Geometry check sheet. Reference: the model listing, model coordinates, mm. A direction names the side the tool comes from. Round coordinates to 2 decimals unless told otherwise and drop trailing zeros. Order: outer loops, then holes, each group sorted by start corner. A loop starts at its lowest first (then second) coordinate and runs counter-clockwise, first axis right, second up.
```python
from build123d import *

# Parameters (mm, degrees)
SKETCH_1_R                   = 7
EXTRUDE_1_DEPTH              = 10
SKETCH_2_R                   = 8
EXTRUDE_2_DEPTH              = 4
SKETCH_3_R                   = 3
EXTRUDE_3_DEPTH              = 9.5
CUT_EXTRUDE_1_DEPTH          = 28.367864531
CUT_EXTRUDE_1_DEPTH_BACK     = 28.367864531
SKETCH_4_R                   = 1
SKETCH_8_R                   = 1
EXTRUDE_4_DEPTH              = 2
HOLE_WIZARD_M5_1_D           = 5.5
HOLE_WIZARD_M5_1_CBORE_D     = 11
HOLE_WIZARD_M5_1_CBORE_DEPTH = 6.5
FILLET_1_R                   = 2


with BuildPart() as part:
    # 草图1 → 凸台-拉伸1 (new body)
    with BuildSketch(Plane(origin=(0, 0, 0), x_dir=(1, 0, 0), z_dir=(0, 1, 0))):
        with Locations(Location((0, 0, 0), (0, 0, 270))):
            Circle(SKETCH_1_R)
    extrude(amount=EXTRUDE_1_DEPTH)

    # 草图2 → 凸台-拉伸2 (add)
    with BuildSketch(Plane(origin=(0, 10, 0), x_dir=(1, 0, 0), z_dir=(0, 1, 0))):
        with Locations(Location((0, 0, 0), (0, 0, 270))):
            Circle(SKETCH_2_R)
    extrude(amount=EXTRUDE_2_DEPTH)

    # 草图3 → 凸台-拉伸3 (add, symmetric)
    with BuildSketch(Plane(origin=(0, 0, 0), x_dir=(0, 0, -1), z_dir=(1, 0, 0))):
        with Locations((0, 15)):
            Circle(SKETCH_3_R)
    extrude(amount=EXTRUDE_3_DEPTH, both=True)

    # 草图4 → 切除-拉伸1 (cut, two sides: drawn at the far end of the back side and taken through both)
    with BuildSketch(Plane(origin=(9.5, 0, 0), x_dir=(0, 0, -1), z_dir=(1, 0, 0)).offset(-CUT_EXTRUDE_1_DEPTH_BACK)):
        with Locations((0, 15)):
            Circle(SKETCH_4_R)
    extrude(amount=CUT_EXTRUDE_1_DEPTH + CUT_EXTRUDE_1_DEPTH_BACK, mode=Mode.SUBTRACT)

    # 草图8 → 凸台-拉伸4 (add, symmetric)
    with BuildSketch(Plane(origin=(0, 0, 0), x_dir=(0, 0, -1), z_dir=(1, 0, 0))):
        Polygon((0, 0), (-20.85568787, 17.5), (-32, 17.5), (-32, 22.5), (-19, 22.5), (0, 7.5), align=None)
        with Locations((-30, 20)):
            Circle(SKETCH_8_R, mode=Mode.SUBTRACT)
        with Locations((-25, 20)):
            Circle(SKETCH_8_R, mode=Mode.SUBTRACT)
    extrude(amount=EXTRUDE_4_DEPTH, both=True)

    # M5 六角头螺栓的柱形沉头孔1 (through all)
    with Locations(Plane(origin=(0, 0, 0), x_dir=(-1, 0, 0), z_dir=(0, -1, 0))):
        with Locations((0, 0)):
            CounterBoreHole(HOLE_WIZARD_M5_1_D / 2, HOLE_WIZARD_M5_1_CBORE_D / 2, HOLE_WIZARD_M5_1_CBORE_DEPTH)

    # 圆角1
    fillet_1_edges = [part.edges().sort_by_distance(p)[0] for p in [
        (0, 22.5, 19),
        (0, 22.5, 32),
        (0, 17.5, 32),
    ]]
    fillet(fillet_1_edges, radius=FILLET_1_R)


solid = part.part
```
(1) Sectioned sample at A-A, the plane z = 0. Record the cut outline in (x, y).
Returned:
outline: (-9.5, 12) - (-8, 12) - (-8, 10) - (-7, 10) - (-7, 0) - (-5.5, 0) - (-5.5, 6.5) - (-2.75, 6.5) - (-2.75, 14) - (-9.5, 14) - close; (-9.5, 16) - (-2.75, 16) - (-2.75, 18) - (-9.5, 18) - close; (2.75, 6.5) - (5.5, 6.5) - (5.5, 0) - (7, 0) - (7, 10) - (8, 10) - (8, 12) - (9.5, 12) - (9.5, 14) - (2.75, 14) - close; (2.75, 16) - (9.5, 16) - (9.5, 18) - (2.75, 18) - close
(2) Set-up check for faces 5 (the cylindrical face through (-6.834, 4.93, -1.517)), 6 (the flat face through (0, 20, 32)): record each of +Z, -Z, +X, -X, +Y, -Y from which the full face is reachable in a straight line by a thin tool's end or side.
Returned:
face 5: -Y
face 6: +Z, +X, -X, +Y, -Y
(3) Depth check by flat-ended pin: P1, Ø1.5, axis at x = 1, z = 11.5, coming from the -Y side; P2, Ø9, axis at x = 0, z = 0, coming from the +Y side; P3, Ø4, axis at x = -2.5, z = 12.5, coming from the -Y side. Enter the tip coordinate at first touch or a pass-through.
Returned:
P1: stops at y = 9.02
P2: stops at y = 18
P3: stops at y = 8.86
(4) Sectioned sample at C-C, the plane x = 1.5. Record the cut outline in (y, z), and give its area (3 significant figures).
Returned:
outline: (0, -6.84) - (10, -6.84) - (10, -7.86) - (14, -7.86) - (14, -2.83) arc R3 ccw to (16.92, -2.3) - (6.5, -2.3) - (6.5, -5.29) - (0, -5.29) - close; (0, 5.29) - (6.5, 5.29) - (6.5, 2.3) - (16.92, 2.3) arc R3 ccw to (14, 2.83) - (14, 7.86) - (13.7, 7.86) - (22.07, 18.46) arc R2 ccw to (22.5, 19.69) - (22.5, 30) arc R2 ccw to (20.5, 32) - (19.5, 32) arc R2 ccw to (17.5, 30) - (17.5, 20.86) - (5.74, 6.84) - (0, 6.84) - close; hole circle Ø2 at (20, 25); hole circle Ø2 at (20, 30)
area: 238 mm2
(5) Material ranges on line 1 (Y direction, x = 7.5, z = 0); line 2 (Z direction, x = 0, y = 4.5); line 3 (X direction, y = 13, z = 2), recorded low to high.
Returned:
line 1: y = 10 to 14, 16 to 18
line 2: z = -7 to -5.5, 5.5 to 7
line 3: x = -9.5 to -1.89, 1.89 to 9.5
(6) Draft check along Y on faces 1 (the flat face through (-9.5, 16, 1)), 2 (the flat face through (-1, 6.5, -3)), 3 (the cylindrical face through (-0.03, 21.93, 31.4)), 4 (the cylindrical face through (-6, 14, 0)). Enter one of: released by +Y, released by -Y, zero draft, split by the parting line, or undercut.
Returned:
face 1: zero draft
face 2: released by -Y
face 3: released by +Y
face 4: undercut
(7) Sectioned sample at B-B, the plane z = 25. Record the cut outline in (x, y).
Returned:
outline: (-2, 17.5) - (2, 17.5) - (2, 19) - (-2, 19) - close; (-2, 21) - (2, 21) - (2, 22.5) - (-2, 22.5) - close
(8) Sectioned sample at D-D, the plane y = 4.5. Record the cut outline in (x, z).
Returned:
outline: circle Ø14 at (0, 0); hole circle Ø11 at (0, 0)
